```python
from build123d import *

# Parameters (mm, degrees)
SKETCH139_R  = 1.8
PAD110_DEPTH = 50
SKETCH125_R  = 3
PAD099_DEPTH = 2
SKETCH123_R  = 1.5
PAD097_DEPTH = 50
PAD083_DEPTH = 6


with BuildPart() as sidemountscrewcutout:
    # Sketch139 → Pad110 (new body, symmetric)
    with BuildSketch(Plane(origin=(0, 34, 0), x_dir=(0, 1, 0), z_dir=(1, 0, 0))):
        with Locations((3.25, 0)):
            Circle(SKETCH139_R)
    extrude(amount=PAD110_DEPTH, both=True)


with BuildPart() as countersinkcutout:
    # Sketch125 → Pad099 (new body)
    with BuildSketch(Plane(origin=(0, 40, 20), x_dir=(1, 0, 0), z_dir=(0, 0, 1))):
        with Locations((0, -3)):
            Circle(SKETCH125_R)
    extrude(amount=PAD099_DEPTH)


with BuildPart() as cutout:
    # Sketch123 → Pad097 (new body)
    with BuildSketch(Plane(origin=(0, 40, 0), x_dir=(1, 0, 0), z_dir=(0, 0, 1))):
        with Locations((0, -3)):
            Circle(SKETCH123_R)
    extrude(amount=PAD097_DEPTH)

    # Fusion004020003: union CountersinkCutout
    add(countersinkcutout.part)


with BuildPart() as motorcagesupportrib:
    # Sketch110 → Pad083 (new body)
    with BuildSketch(Plane.XZ.offset(-40)):
        Polygon((-23, -11.252777), (-23, 11.252777), (-10.252777, 24), (10.252777, 24), (23, 11.252777), (23, -11.252777), (20, -9.520726), (20, 8.284271), (8.284271, 20), (-8.284271, 20), (-20, 8.284271), (-20, -9.520726), align=None)
    extrude(amount=PAD083_DEPTH)

    # Cut007019008: cut Cutout
    add(cutout.part, mode=Mode.SUBTRACT)


with BuildPart() as motorcagesupportrib_1:
    # Cut007019008 placement: moved
    add(motorcagesupportrib.part.moved(Location((0, 0.25, 0))))

    # Cut007019012: cut SideMountScrewCutout
    add(sidemountscrewcutout.part, mode=Mode.SUBTRACT)


solid = motorcagesupportrib_1.part
```
Model file for the job. Use its own axes, mm. A direction names the side the tool comes from. Round coordinates to 2 decimals unless told otherwise and drop trailing zeros. Write each loop counter-clockwise with the first axis right and the second up, starting at its lowest first coordinate (ties: lowest second). Pieces come first, ordered by that corner, then holes. Notation, with made-up numbers: (21.25, -25.75) - (48.25, -25.75) arc R15 cw to (48.25, -13.75) - close; hole circle Ø6 at (3, 65.5). An arc over 180 degrees is marked (long way). Use CSV: the item, a comma, the result in double quotes. Start each with the question number.
Item 1: Drill centre lines: L1, parallel to Y at x = 0, z = 23.55; L2, parallel to X at y = 35.05, z = 8; L3, parallel to Z at x = -5, y = 37. Where is each one in solid material? Low to high. Write a range as [from, to].
Item 2: Band-saw the part on D-D (y = 37.25). Write the cut outline in (x, z).
Item 3: Band-saw the part on B-B (y = 34.85). Write the cut outline in (x, z).
Item 4: Tool access for faces 1 (the face through (-3, 37.3, 21)), 2 (the face through (-2, 40.25, 21)), 3 (the face through (5, 37, 20)): list every direction of +Z, -Z, +X, -X, +Y, -Y with a clear straight run to the whole face (end or side of a thin tool).
Item 5: Pin check, flat tips, straight feed: P1, Ø2, axis at y = 38, z = 19.5, coming from the +X side; P2, Ø2, axis at y = 37.5, z = 19.5, coming from the -X side. Stop position of each tip, or through.
Item 6: Two-plate mould, pull along Y, no slides. Class faces 4 (the face through (1, 39, 22)), 5 (the face through (-2, 34.25, 21)), 6 (the face through (16.537, 37.292, 17.716)): released by +Y, released by -Y, zero draft, split by the parting line, or undercut.
Item 7: Band-saw the part on C-C (z = 0). Write the cut outline in (x, y).
Item 8: Band-saw the part on A-A (z = -7). Write the cut outline in (x, y), and give its area (3 significant figures).
Checked values:
1,L1,"y = [34.25, 35.75], [38.75, 40.25]"
1,L2,"x = [-23, -20], [20, 23]"
1,L3,"z = [20, 24]"
2,outline,"(-23, -11.25) - (-20, -9.52) - (-20, -1.8) - (-23, -1.8) - close; (-23, 1.8) - (-20, 1.8) - (-20, 8.28) - (-8.28, 20) - (-3, 20) - (-3, 22) - (-1.5, 22) - (-1.5, 24) - (-10.25, 24) - (-23, 11.25) - close; (1.5, 22) - (3, 22) - (3, 20) - (8.28, 20) - (20, 8.28) - (20, 1.8) - (23, 1.8) - (23, 11.25) - (10.25, 24) - (1.5, 24) - close; (20, -9.52) - (23, -11.25) - (23, -1.8) - (20, -1.8) - close"
3,outline,"(-23, -11.25) - (-20, -9.52) - (-20, 8.28) - (-8.28, 20) - (-1.8, 20) - (-1.8, 22) - (1.8, 22) - (1.8, 20) - (8.28, 20) - (20, 8.28) - (20, -9.52) - (23, -11.25) - (23, 11.25) - (10.25, 24) - (-10.25, 24) - (-23, 11.25) - close"
4,face 1,"-Z"
4,face 2,"+Z, -Z, +X, -X, +Y"
4,face 3,"-Z, +Y, -Y"
5,P1,"stops at x = 15.75"
5,P2,"stops at x = -15.75"
6,face 4,"undercut"
6,face 5,"released by -Y"
6,face 6,"zero draft"
7,outline,"(-23, 34.25) - (-20, 34.25) - (-20, 35.45) - (-23, 35.45) - close; (-23, 39.05) - (-20, 39.05) - (-20, 40.25) - (-23, 40.25) - close; (20, 34.25) - (23, 34.25) - (23, 35.45) - (20, 35.45) - close; (20, 39.05) - (23, 39.05) - (23, 40.25) - (20, 40.25) - close"
8,outline,"(-23, 34.25) - (-20, 34.25) - (-20, 40.25) - (-23, 40.25) - close; (20, 34.25) - (23, 34.25) - (23, 40.25) - (20, 40.25) - close"
8,area,"36.0 mm²"
